```python
from build123d import *
from build123d.topology import SkipClean

# Parameters (mm, degrees)
ESQUISSE2_W             = 24.25
ESQUISSE2_H             = 13.2
ESQUISSE2_R             = 0.5
BOSS_EXTRU_1_DEPTH      = 9.3
ESQUISSE3_W             = 24.25
ESQUISSE3_H             = 13.2
ESQUISSE3_R             = 2.45
ESQUISSE3_R_2           = 0.75
BOSS_EXTRU_2_DEPTH      = 1
ESQUISSE4_R             = 1
ENL_V_MAT_EXTRU_1_DEPTH = 29.992455915
ESQUISSE5_W             = 13.8
ESQUISSE5_H             = 1
BOSS_EXTRU_3_DEPTH      = 13.8
CONG_1_R                = 5
BOSS_EXTRU_4_START      = 1.8
ESQUISSE8_R             = 3.45
ESQUISSE8_R_2           = 2.45
BOSS_EXTRU_4_DEPTH      = 1.8
ESQUISSE9_R             = 0.7
ENL_V_MAT_EXTRU_2_DEPTH = 8


with BuildPart() as part:
    # Esquisse2 → Boss.-Extru.1 (new body)
    with BuildSketch(Plane(origin=(0, 0, 0), x_dir=(1, 0, 0), z_dir=(0, 1, 0))):
        with Locations((11.025, 5.5)):
            Rectangle(ESQUISSE2_W, ESQUISSE2_H)
        Polygon((0, 8.5), (2.5, 11), (19.55, 11), (22.05, 8.5), (22.05, 2.5), (19.55, 0), (2.5, 0), (0, 2.5), align=None, mode=Mode.SUBTRACT)
        with Locations(Location((0.5, 10.5, 0), (0, 0, 270))):
            Circle(ESQUISSE2_R, mode=Mode.SUBTRACT)
        with Locations(Location((21.55, 10.5, 0), (0, 0, 270))):
            Circle(ESQUISSE2_R, mode=Mode.SUBTRACT)
        with Locations(Location((0.5, 0.5, 0), (0, 0, 270))):
            Circle(ESQUISSE2_R, mode=Mode.SUBTRACT)
        with Locations(Location((21.55, 0.5, 0), (0, 0, 270))):
            Circle(ESQUISSE2_R, mode=Mode.SUBTRACT)
    extrude(amount=BOSS_EXTRU_1_DEPTH)

    # Esquisse3 → Boss.-Extru.2 (add)
    with BuildSketch(Plane(origin=(0, 9.3, 0), x_dir=(1, 0, 0), z_dir=(0, 1, 0))):
        with Locations((11.025, 5.5)):
            Rectangle(ESQUISSE3_W, ESQUISSE3_H)
        with Locations(Location((6, 5.5, 0), (0, 0, 270))):
            Circle(ESQUISSE3_R, mode=Mode.SUBTRACT)
        with Locations(Location((12, 5.5, 0), (0, 0, 270))):
            Circle(ESQUISSE3_R_2, mode=Mode.SUBTRACT)
    extrude(amount=BOSS_EXTRU_2_DEPTH)

    # Esquisse4 → Enlèv. mat.-Extru.1 (cut, through all)
    with BuildSketch(Plane(origin=(23.15, 0, 0), x_dir=(0, 0, -1), z_dir=(1, 0, 0))):
        with Locations((5.5, 5.8)):
            Circle(ESQUISSE4_R)
    extrude(amount=-ENL_V_MAT_EXTRU_1_DEPTH, mode=Mode.SUBTRACT)

    # Esquisse5 → Révolution1 (revolve)
    with BuildSketch(Plane.XY.offset(-5.5), mode=Mode.PRIVATE) as r_volution1_sk:
        with Locations((-8, 6.8)):
            Rectangle(ESQUISSE5_W, ESQUISSE5_H)
        Polygon((22.05, 10.3), (22.05, 5.8), (26.15, 5.8), (26.15, 8.2), (29.15, 8.2), (29.15, 10.3), align=None)
    revolve(r_volution1_sk.sketch.rotate(Axis((-19.031616201, 5.8, -5.5), (1, 0, 0)), 90), axis=Axis((-19.031616201, 5.8, -5.5), (1, 0, 0)))

    # Esquisse6 → Boss.-Extru.3 (add)
    with BuildSketch(Plane.ZY.offset(14.9)):
        with BuildLine():
            Line((-7, 5.8), (-7, 10.3))
            Line((-7, 10.3), (-4, 10.3))
            Line((-4, 10.3), (-4, 5.8))
            ThreePointArc((-4, 5.8), (-5.5, 7.3), (-7, 5.8))
        make_face()
    extrude(amount=-BOSS_EXTRU_3_DEPTH)

    # Congé1
    cong_1_edges = [part.edges().sort_by_distance(p)[0] for p in [
        (-1.1, 8.05, -4),
        (-1.1, 8.05, -7),
        (-1.1, 4.3, -5.5),
    ]]
    fillet(cong_1_edges, radius=CONG_1_R)

    # Esquisse8 → Boss.-Extru.4 (add)
    with SkipClean():  # the faces are left unmerged after this step: merging them gives an invalid solid
        with BuildSketch(Plane.XZ.offset(-9.3).offset(BOSS_EXTRU_4_START)):
            with Locations(Location((6, -5.5, 0), (0, 0, 90))):
                Circle(ESQUISSE8_R)
            with Locations(Location((6, -5.5, 0), (0, 0, 270))):
                Circle(ESQUISSE8_R_2, mode=Mode.SUBTRACT)
        extrude(amount=-BOSS_EXTRU_4_DEPTH)

    # Esquisse9 → Enlèv. mat.-Extru.2 (cut)
    with SkipClean():  # the faces are left unmerged after this step: merging them gives an invalid solid
        with BuildSketch(Plane.ZY.offset(14.9)):
            with Locations((-5.5, 5.8)):
                Circle(ESQUISSE9_R)
        extrude(amount=-ENL_V_MAT_EXTRU_2_DEPTH, mode=Mode.SUBTRACT)


solid = part.part
```
Geometry check sheet. Reference: the model listing, model coordinates, mm. A direction names the side the tool comes from. Coordinates: 2 decimals unless noted, no trailing zeros. Order: outer loops, then holes, each group sorted by start corner. A loop starts at its lowest first (then second) coordinate and runs counter-clockwise, first axis right, second up. Notation, with made-up numbers: (28.25, 5.5) - (62.25, 5.5) arc R20 cw to (62.25, 26.5) - close; hole circle Ø9 at (16.5, -25). An arc over 180 degrees is marked (long way). Answer in a Markdown table with one row per item. Add a question column.
1. Gauge pin test, flat ends, axial feed: pin 1 Ø0.8 at (y, z) = (5.8, -5.5) entering from -X; pin 2 Ø2 at (y, z) = (6, -5.5) entering from +X; pin 3 Ø2.5 at (x, y) = (-10.5, 8) entering from -Z; pin 4 Ø2 at (x, z) = (-6, -9) entering from +Y. Record the tip position at first contact, or that the pin passes through.
2. Section check B-B (x = -12). Enter the section's corners in (y, z), plus the area to 3 significant figures.
3. Section check D-D (y = 2.5). Give the number of separate pieces and of enclosed holes in the cut face, plus the area to 3 significant figures.
4. Section check C-C (x = 0.5). Enter the section's corners in (y, z), plus the area to 3 significant figures.
5. Access from +Z, -Z, +X, -X, +Y, -Y to the whole of each face (thin tool, end or side, straight path). Record for faces 4 (the face through (-1.1, 2, -11)), 5 (the face through (-10.4, 4.3, -5.5)), 6 (the face through (26.11, 1.34, -6.09)), 7 (the face through (-11, 8, -4)), 8 (the face through (1.3, 4.6, -1.2)).
6. Material ranges on L1, parallel to Z at x = 8, y = 1.75; L2, parallel to X at y = 9.8, z = -5.5; L3, parallel to X at y = 3.5, z = -0.5, recorded low to high. Write a range as [from, to].
7. Draft check along X on faces 1 (the face through (8.1, 10.3, -7.1)), 2 (the face through (11, 5, -11)), 3 (the face through (-2.53, 8.02, -2.5)). Enter one of: +X half, -X half, draft (parallel to the pull), parting line (faces both ways), or undercut.
Data:
| question | item | result |
|---|---|---|
| 1 | pin 1 | stops at x = 22.05 |
| 1 | pin 2 | stops at x = 26.15 |
| 1 | pin 3 | stops at z = -7 |
| 1 | pin 4 | passes through |
| 2 | outline | (5.8, -7) - (10.3, -7) - (10.3, -4) - (5.8, -4) arc R1.5 ccw to start; hole circle Ø1.4 at (5.8, -5.5) |
| 2 | area | 15.5 mm² |
| 3 | separate pieces | 1 |
| 3 | enclosed holes | 5 |
| 3 | area | 130 mm² |
| 4 | outline | (0, -12.1) - (10.3, -12.1) - (10.3, 1.1) - (0, 1.1) - (0, 0) - (9.3, 0) - (9.3, -1) - (0, -1) - (0, -2) - (9.3, -2) - (9.3, -9) - (0, -9) - (0, -10) - (9.3, -10) - (9.3, -11) - (0, -11) - close |
| 4 | area | 52.3 mm² |
| 5 | face 4 | -Z, -X, -Y |
| 5 | face 5 | -X, -Y |
| 5 | face 6 | +X |
| 5 | face 7 | +Z, -X, +Y, -Y |
| 5 | face 8 | -Y |
| 6 | L1 | z = [-12.1, -11], [0, 1.1] |
| 6 | L2 | x = [-14.9, 3.55], [8.45, 11.25], [12.75, 29.15] |
| 6 | L3 | x = [-1.2, 0], [1, 2], [20.05, 21.05], [22.05, 23.15] |
| 7 | face 1 | draft |
| 7 | face 2 | undercut |
| 7 | face 3 | -X half |
